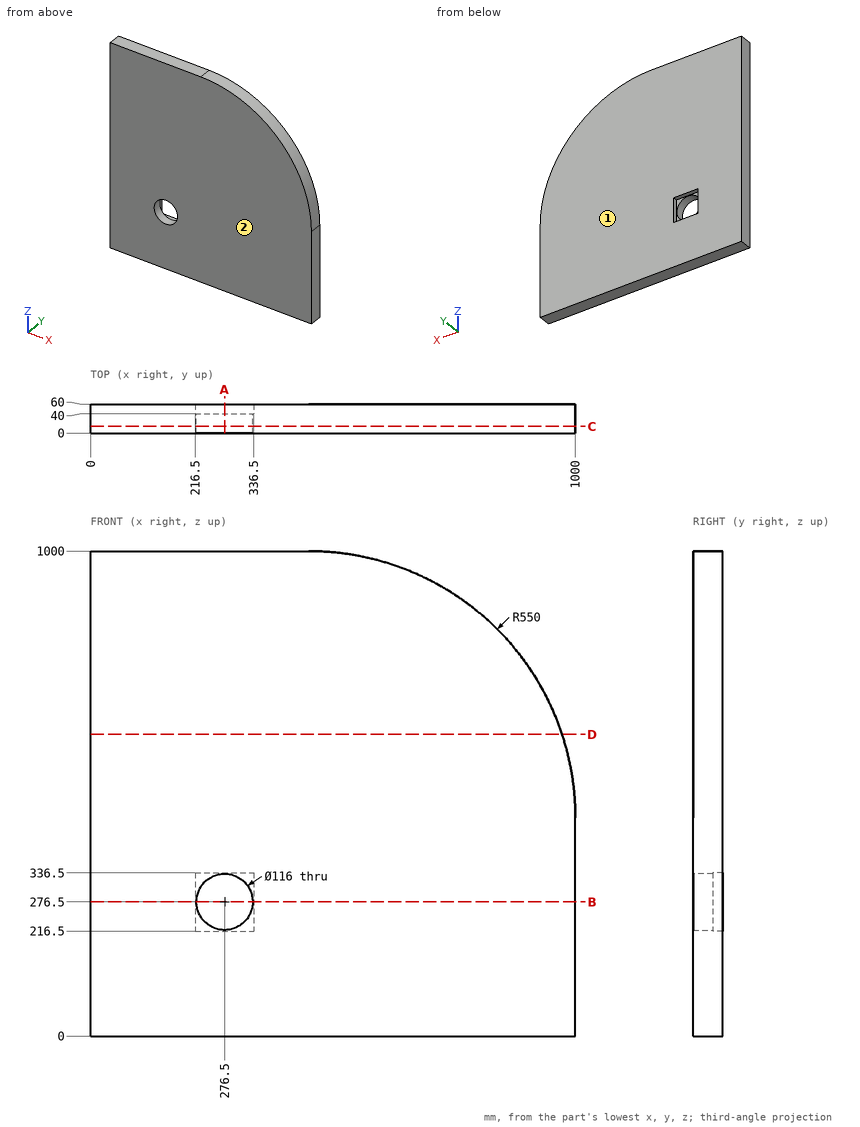
Job drawing, mm, ordinate dimensions from the low corner. One solid piece. Give positions to 0.01 mm unless a question says otherwise; leave off trailing zeros. Loops run counter-clockwise (first coordinate to the right, second up) from the corner with the lowest first, then second, coordinate; pieces in that order, holes last. Notation, with made-up numbers: (85, 76) -> (95, 76) arc R16 cw to (95, 82) -> close; hole circle Ø10 at (28.5, -28). An arc over 180 degrees is marked (long way). Write each question's results on one line, items separated by ' | '.
(1) Probe line 1 along Z through (x, y) = (276, 30); line 2 along Z through (x, y) = (285.5, 41); line 3 along X through (y, z) = (23.5, 292.5). List the from-to ranges inside material, lowest first.
Geometry results:
line 1: z = 0 to 218.5, 334.5 to 1000 | line 2: z = 0 to 216.5, 336.5 to 1000 | line 3: x = 0 to 220.75, 332.25 to 1000
(2) Pull direction Y, two halves, no side cores. Call the marked faces 1 and 2: released by +Y, released by -Y, zero draft, split by the parting line, or undercut.
Geometry results:
face 1: released by +Y | face 2: released by -Y
(3) Cut at B-B on z = 276.5. List the corners of the cut face in (x, y).
Geometry results:
outline: (0, 0) -> (218.5, 0) -> (218.5, 40) -> (216.5, 40) -> (216.5, 60) -> (0, 60) -> close; (334.5, 0) -> (1000, 0) -> (1000, 60) -> (336.5, 60) -> (336.5, 40) -> (334.5, 40) -> close
(4) Cut at C-C on y = 14. List the corners of the cut face in (x, z), and give its area (3 significant figures).
Geometry results:
outline: (0, 0) -> (1000, 0) -> (1000, 450) arc R550 ccw to (450, 1000) -> (0, 1000) -> close; hole circle Ø116 at (276.5, 276.5) | area: 925,000 mm²
(5) Cut at D-D on z = 622. List the corners of the cut face in (x, y), and give its area (3 significant figures).
Geometry results:
outline: (0, 0) -> (972.41, 0) -> (972.41, 60) -> (0, 60) -> close | area: 58,300 mm²
(6) Flat gauge pin, fed straight in: pin 1 Ø1.5 at (x, y) = (634, 41) entering from +Z. Where does the tip first touch, or does it go through?
Geometry results:
pin 1: stops at z = 968.57
(7) Cut at A-A on x = 276.5. List the corners of the cut face in (y, z).
Geometry results:
outline: (0, 0) -> (60, 0) -> (60, 216.5) -> (40, 216.5) -> (40, 218.5) -> (0, 218.5) -> close; (0, 334.5) -> (40, 334.5) -> (40, 336.5) -> (60, 336.5) -> (60, 1000) -> (0, 1000) -> close
